```python
from build123d import *

# Parameters (mm, degrees)
SKETCH_1_R            = 2.75
EXTRUDE_248_DEPTH     = 3
CUT_EXTRUDE_378_DEPTH = 1.3
SKETCH_3_R            = 1.5
EXTRUDE_479_DEPTH     = 55


with BuildPart() as part:
    # 草图1 → Extrude 248 (new body)
    with BuildSketch(Plane(origin=(0, 0, 0), x_dir=(1, 0, 0), z_dir=(0, 1, 0))):
        Circle(SKETCH_1_R)
    extrude(amount=EXTRUDE_248_DEPTH)

    # 草图2 → Cut-Extrude 378 (cut)
    with BuildSketch(Plane(origin=(0, 3, 0), x_dir=(1, 0, 0), z_dir=(0, 1, 0))):
        Polygon((1.443375673, 0), (0.721687836, 1.25), (-0.721687836, 1.25), (-1.443375673, 0), (-0.721687836, -1.25), (0.721687836, -1.25), align=None)
    extrude(amount=-CUT_EXTRUDE_378_DEPTH, mode=Mode.SUBTRACT)

    # 草图3 → Extrude 479 (add)
    with BuildSketch(Plane.XZ):
        Circle(SKETCH_3_R)
    extrude(amount=EXTRUDE_479_DEPTH)


solid = part.part
```
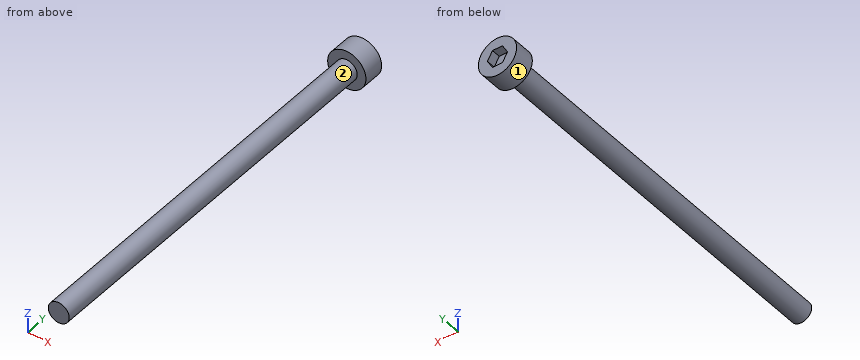
Source: CAD feature listing. Evaluate the final solid. Frame: model axes, mm. Face numbers are marked on the shaded views. A direction names the side the tool comes from. Round coordinates to 2 decimals unless told otherwise and drop trailing zeros. Loops run counter-clockwise (first coordinate to the right, second up) from the corner with the lowest first, then second, coordinate; pieces in that order, holes last. Notation, with made-up numbers: M -35,-30.5 L -20,-30.5 A13 cw -20,-15.5 Z; hole C 80,-23.75 d10. An arc over 180 degrees is marked long. Use a Markdown table: item, result. Add a question column.
1. Contact query for flat-ended pins moving along their axis: P1, Ø1, axis at y = -47, z = 1.5, coming from the -X side; P2, Ø3, axis at y = -47, z = 0.5, coming from the +X side; P3, Ø0.8, axis at x = 0, z = 0, coming from the +Y side. Output: stop coordinate, or through.
2. Section query A-A on x = 0. Return the cut outline in (y, z).
3. Line query: line 1 (Y direction, x = -0.45, z = 0.95); line 2 (Y direction, x = -0.2, z = -1.65); line 3 (X direction, y = -50.5, z = 0.15). Output: solid intervals per line, ascending.
4. Section query B-B on y = -24.5. Return the cut outline in (x, z).
5. Reachability of the marked faces 1 and 2 from +Z, -Z, +X, -X, +Y, -Y: full face, straight path, thin tool, end or side. Return the list, or none.
Reported:
| question | item | result |
|---|---|---|
| 1 | P1 | stops at x = -1.12 |
| 1 | P2 | stops at x = 1.5 |
| 1 | P3 | stops at y = 1.7 |
| 2 | outline | M -55,-1.5 L 0,-1.5 L 0,-2.75 L 3,-2.75 L 3,-1.25 L 1.7,-1.25 L 1.7,1.25 L 3,1.25 L 3,2.75 L 0,2.75 L 0,1.5 L -55,1.5 Z |
| 3 | line 1 | y = -55 to 1.7 |
| 3 | line 2 | y = 0 to 3 |
| 3 | line 3 | x = -1.49 to 1.49 |
| 4 | outline | C 0,0 d3 |
| 5 | face 1 | +Y, -Y |
| 5 | face 2 | -Y |
